Could you check a few things on this drawing? It's one solid part, dimensions in mm from its lowest x, y, z. Round coordinates to 2 decimals unless told otherwise and drop trailing zeros. Loops run counter-clockwise (first coordinate to the right, second up) from the corner with the lowest first, then second, coordinate; pieces in that order, holes last. Notation, with made-up numbers: M 74,72.5 L 111,72.5 A35 cw 111,111.5 Z; hole C -38.75,-37.5 d5. An arc over 180 degrees is marked long. Write each question's results on one line, items separated by ' | '. Start each with the question number.
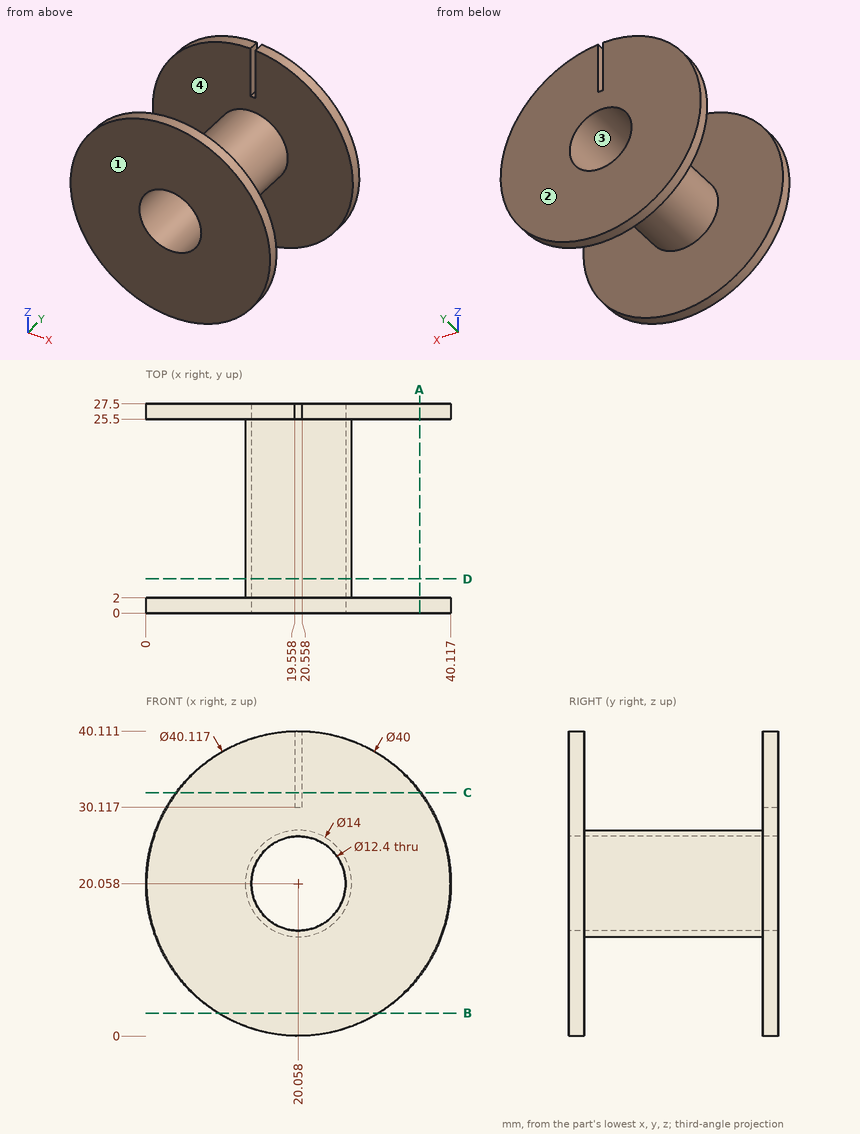
1. I want a section at A-A on x = 36. List the corners of the cut face in (y, z) for me (1 decimal).
2. For pin 1 (1.6 mm diameter, centred on y = 26.5, z = 37, fed in from +X) (1 decimal); pin 2 (1.6 mm diameter, centred on y = 26.5, z = 34.5, fed in from -X); pin 3 (10 mm diameter, centred on y = 21, z = 4, fed in from -X) (1 decimal), each with a flat end and sliding along its axis, tell me the tip position at first contact or that it passes through.
3. I want a section at B-B on z = 3. List the corners of the cut face in (x, y) for me.
4. I want a section at D-D on y = 4.5. List the corners of the cut face in (x, z) for me.
5. If we mould it in two halves opening along Y, with no side actions, what happens to the marked faces 1, 2, 3 and 4? For each: released by +Y, released by -Y, zero draft, split by the parting line, or undercut.
6. I need wall thicknesses on line 1 along Y through (x, z) = (11, 13); line 2 along X through (y, z) = (10.5, 23) (1 decimal); line 3 along Z through (x, y) = (24, 23) (1 decimal). Which ranges of each line are inside material? Lowest first, please.
7. I want a section at C-C on z = 32. List the corners of the cut face in (x, y) for me (1 decimal), plus the area to 3 significant figures.
Outcome:
1) outline: M 0,8 L 2,8 L 2,32.1 L 0,32.1 Z; M 25.5,7.9 L 27.5,7.9 L 27.5,32.2 L 25.5,32.2 Z
2) pin 1: x = 32 | pin 2: x = 5.35 | pin 3: x = 5.6
3) outline: M 9.51,25.5 L 30.61,25.5 L 30.61,27.5 L 9.51,27.5 Z; M 9.62,0 L 30.5,0 L 30.5,2 L 9.62,2 Z
4) outline: C 20.06,20.06 d14; hole C 20.06,20.06 d12.4
5) face 1: released by -Y | face 2: released by +Y | face 3: zero draft | face 4: undercut
6) line 1: 0 to 2, 25.5 to 27.5 | line 2: 13.7 to 14.6, 25.5 to 26.4 | line 3: 14.3 to 15.3, 24.8 to 25.8
7) outline: M 3.9,25.5 L 19.6,25.5 L 19.6,27.5 L 3.9,27.5 Z; M 4,0 L 36.1,0 L 36.1,2 L 4,2 Z; M 20.6,25.5 L 36.2,25.5 L 36.2,27.5 L 20.6,27.5 Z | area: 127 mm2
